from build123d import *


with BuildPart() as part:
    # Esquisse1 → Révolution1 (revolve)
    with BuildSketch(Plane.XY, mode=Mode.PRIVATE) as r_volution1_sk:
        with BuildLine():
            Line((1.981656821, 8.97797736), (7.823456821, 8.97797736))
            Line((7.823456821, 8.97797736), (4.683813218, 2.298439639))
            ThreePointArc((4.683813218, 2.298439639), (3.207806254, 0.623149289), (1.06377284, 0))
            Line((1.06377284, 0), (0.803456821, 0))
            Line((0.803456821, 0), (-5.036543179, 0))
            Line((-5.036543179, 0), (-15.076543179, 1.81597736))
            Line((-15.076543179, 1.81597736), (-15.076543179, 4.15197736))
            Line((-15.076543179, 4.15197736), (-2.000513414, 4.15197736))
            ThreePointArc((-2.000513414, 4.15197736), (-1.65849327, 4.212284739), (-1.357725804, 4.385932917))
            Line((-1.357725804, 4.385932917), (-0.12815557, 5.417664847))
            ThreePointArc((-0.12815557, 5.417664847), (0.135364608, 5.761091028), (0.229056821, 6.18370929))
            Line((0.229056821, 6.18370929), (0.229056821, 7.34597736))
            Line((0.229056821, 7.34597736), (1.981656821, 7.34597736))
            Line((1.981656821, 7.34597736), (1.981656821, 8.97797736))
        make_face()
    revolve(r_volution1_sk.sketch.rotate(Axis((-19.476947674, -3.82202264, 0), (1, 0, 0)), 90), axis=Axis((-19.476947674, -3.82202264, 0), (1, 0, 0)))


solid = part.part
Geometry check sheet. Reference: the model listing, model coordinates, mm. A direction names the side the tool comes from. Give positions to 0.01 mm unless a question says otherwise; leave off trailing zeros. Order: outer loops, then holes, each group sorted by start corner. A loop starts at its lowest first (then second) coordinate and runs counter-clockwise, first axis right, second up. Notation, with made-up numbers: M 40,-38 L 79,-38 A20 ccw 79,-31 Z; hole C 14.5,51.25 d8. An arc over 180 degrees is marked long. Use a Markdown table: item, result.
Item 1: Material ranges on line 1 along Z through (x, y) = (-1, -3.25); line 2 along Z through (x, y) = (-6.5, -2.75); line 3 along Y through (x, z) = (-1.5, 0), recorded low to high.
Answers follow:
| item | result |
|---|---|
| line 1 | z = -8.49 to -3.78, 3.78 to 8.49 |
| line 2 | z = -7.9 to -3.94, 3.94 to 7.9 |
| line 3 | y = -11.93 to -7.64, 0 to 4.29 |
Item 2: Section check B-B (x = -0.75). Record the cut outline in (y, z).
Answers follow:
| item | result |
|---|---|
| outline | C -3.82,0 d17.44; hole C -3.82,0 d7.64 |
Item 3: Draft check along Y on faces 3 (the cylindrical face through (1.118, -14.895, -1.454)), 4 (the flat face through (-15.077, 1.4, -3.4)), 5 (the cylindrical face through (-2.03, -0.09, -0.83)). Enter one of: +Y half, -Y half, draft (parallel to the pull), parting line (faces both ways), or undercut.
Answers follow:
| item | result |
|---|---|
| face 3 | parting line |
| face 4 | draft |
| face 5 | undercut |
Item 4: Tool access check on faces 1 (the cylindrical face through (-8.447, -10.546, 4.287)), 2 (the cylindrical face through (4.9, -7.7, 12.2)). Record the directions out of +Z, -Z, +X, -X, +Y, -Y that give a thin tool (end or side, any length) a straight path to the whole face; none if there is none.
Answers follow:
| item | result |
|---|---|
| face 1 | -X |
| face 2 | +X, -X |
Item 5: Depth check by flat-ended pin: P1, Ø3, axis at x = -9, z = 0, coming from the +Y side; P2, Ø1.5, axis at y = -10, z = -9, coming from the -X side; P3, Ø8, axis at x = -2.5, y = -0.5, coming from the -Z side. Enter the tip coordinate at first touch or a pass-through.
Answers follow:
| item | result |
|---|---|
| P1 | stops at y = 4.15 |
| P2 | stops at x = 0.23 |
| P3 | stops at z = -11.16 |
Item 6: Section check A-A (z = 0). Record the cut outline in (x, y).
Answers follow:
| item | result |
|---|---|
| outline | M -15.08,-11.8 L -2,-11.8 A1 cw -1.36,-12.03 L -0.13,-13.06 A1 cw 0.23,-13.83 L 0.23,-14.99 L 1.98,-14.99 L 1.98,-16.62 L 7.82,-16.62 L 4.68,-9.94 A4 ccw 1.06,-7.64 L -5.04,-7.64 L -15.08,-9.46 Z; M -15.08,1.82 L -5.04,0 L 1.06,0 A4 ccw 4.68,2.3 L 7.82,8.98 L 1.98,8.98 L 1.98,7.35 L 0.23,7.35 L 0.23,6.18 A1 cw -0.13,5.42 L -1.36,4.39 A1 cw -2,4.15 L -15.08,4.15 Z |
